```python
from build123d import *

# Parameters (mm, degrees)
F0_W     = 92
F0_H     = 79
F0_R     = 19.352755
F1_DEPTH = 1
F2_W     = 92
F2_H     = 1
F3_DEPTH = 1


with BuildPart() as f1:
    # F0 (on Front) → F1 (new body)
    with BuildSketch(Plane.XZ):
        Rectangle(F0_W, F0_H)
        Circle(F0_R, mode=Mode.SUBTRACT)
    extrude(amount=F1_DEPTH)

    # F2 (on face) → F3 (join)
    with BuildSketch(Plane.XZ.offset(1)):
        with Locations((0, 36)):
            Rectangle(F2_W, F2_H)
        with Locations((0, -36)):
            Rectangle(F2_W, F2_H)
    extrude(amount=F3_DEPTH)


solid = f1.part
```
Source: CAD feature listing. Evaluate the final solid. Frame: model axes, mm. A direction names the side the tool comes from. Coordinates: 2 decimals unless noted, no trailing zeros. Loops run counter-clockwise (first coordinate to the right, second up) from the corner with the lowest first, then second, coordinate; pieces in that order, holes last. Notation, with made-up numbers: M 21.5,82.25 L 51.5,82.25 A27 ccw 51.5,103.25 Z; hole C 68,70 d2. An arc over 180 degrees is marked long. Put each result on its own line as item: value. Start each with the question number.
1) Cut plane B-B on y = -1.45. Return the cut outline in (x, z).
2) Cut plane A-A on z = 0. Return the cut outline in (x, y), then the cut area to 3 significant figures.
3) Pull-direction query (Z, two-part tool) for faces 3 (the face through (-10.9, -1, 16.3)), 4 (the face through (-1, -1, 38)); classes: pulls with the +Z half, pulls with the -Z half, needs draft (parallel to the pull), parting line crosses it, or undercut.
4) Cut plane D-D on x = 39. Return the cut outline in (y, z).
5) Ray query, L1, parallel to Z at x = 3.5, y = -1.9; L2, parallel to Y at x = 3, z = -33; L3, parallel to X at y = -0.05, z = -6. Return the intervals inside material, ascending. Write a range as from..to.
6) Reachability of faces 1 (the face through (-11, 0, 18)), 2 (the face through (-1, -1, -38)) from +Z, -Z, +X, -X, +Y, -Y: full face, straight path, thin tool, end or side. Return the list, or none.
7) Contact query for flat-ended pins moving along their axis: pin 1 Ø0.5 at (x, y) = (-3, -1.5) entering from +Z; pin 2 Ø8 at (x, z) = (-7, 14.5) entering from -Y; pin 3 Ø0.5 at (x, y) = (-5.5, -1.5) entering from -Z. Output: stop coordinate, or through.
8) Cut plane C-C on x = 0. Return the cut outline in (y, z).
The answers:
1. outline: M -46,-36.5 L 46,-36.5 L 46,-35.5 L -46,-35.5 Z; M -46,35.5 L 46,35.5 L 46,36.5 L -46,36.5 Z
2. outline: M -46,-1 L -19.35,-1 L -19.35,0 L -46,0 Z; M 19.35,-1 L 46,-1 L 46,0 L 19.35,0 Z
2. area: 53.3 mm²
3. face 3: undercut
3. face 4: needs draft
4. outline: M -2,-36.5 L -1,-36.5 L -1,-39.5 L 0,-39.5 L 0,39.5 L -1,39.5 L -1,36.5 L -2,36.5 L -2,35.5 L -1,35.5 L -1,-35.5 L -2,-35.5 Z
5. L1: z = -36.5..-35.5, 35.5..36.5
5. L2: y = -1..0
5. L3: x = -46..-18.4, 18.4..46
6. face 1: +Z, -Z, +X, -X, +Y
6. face 2: -Z, +X, -X, -Y
7. pin 1: stops at z = 36.5
7. pin 2: stops at y = -1
7. pin 3: stops at z = -36.5
8. outline: M -2,-36.5 L -1,-36.5 L -1,-39.5 L 0,-39.5 L 0,-19.35 L -1,-19.35 L -1,-35.5 L -2,-35.5 Z; M -2,35.5 L -1,35.5 L -1,19.35 L 0,19.35 L 0,39.5 L -1,39.5 L -1,36.5 L -2,36.5 Z
